Answer from the drawing. Dimensions are ordinates in mm from the lowest x, y and z of the part. A direction names the side the tool comes from. Give positions to 0.01 mm unless a question says otherwise; leave off trailing zeros. Write each loop counter-clockwise with the first axis right and the second up, starting at its lowest first coordinate (ties: lowest second). Pieces come first, ordered by that corner, then holes.
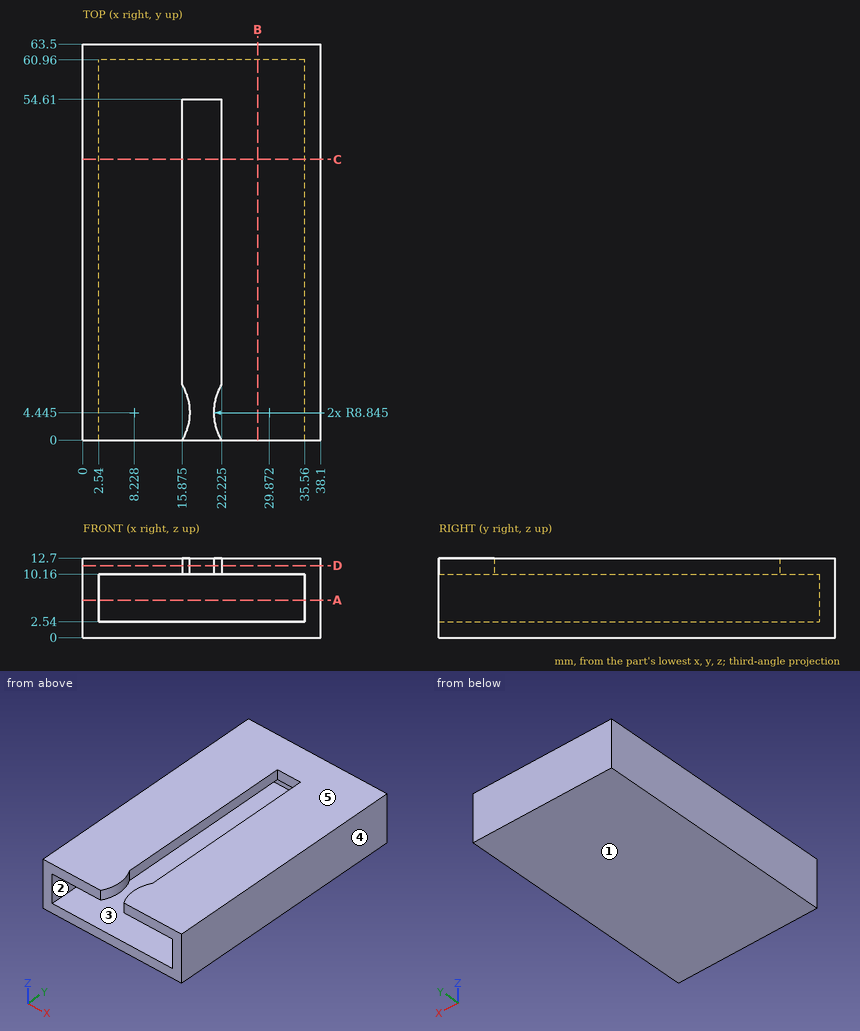
Item 1: Which of the six approach directions +Z, -Z, +X, -X, +Y, -Y give full straight-line access (tool end or side, diameter ignored) to the marked faces 1 and 2?
Result set:
face 1: -Z, +X, -X, +Y, -Y
face 2: -Y
Item 2: Section D-D (z = 11.5) is taken. Write down the section's boundary in (x, y) (1 decimal), and give its area (3 significant figures).
Result set:
outline: (0, 0) - (15.9, 0) arc R8.8 ccw to (15.9, 8.9) - (15.9, 54.6) - (22.2, 54.6) - (22.2, 8.9) arc R8.8 ccw to (22.2, 0) - (38.1, 0) - (38.1, 63.5) - (0, 63.5) - close
area: 2,090 mm2
Item 3: Each of these flat-tipped pins is pushed along its axis until it touches: pin 1 Ø1.3 at (x, z) = (18.5, 11.5) entering from -Y; pin 2 Ø6 at (x, z) = (30.5, 6) entering from -Y. Where does it stop, or does it pass through?
Result set:
pin 1: stops at y = 54.61
pin 2: stops at y = 60.96
Item 4: Determine the mould class of the marked faces 3, 4 and 5 for opening direction Z: pulls with the +Z half, pulls with the -Z half, needs draft (parallel to the pull), parting line crosses it, or undercut.
Result set:
face 3: undercut
face 4: needs draft
face 5: pulls with the +Z half
Item 5: Section B-B (x = 28) is taken. Write down the section's boundary in (y, z).
Result set:
outline: (0, 0) - (63.5, 0) - (63.5, 12.7) - (0, 12.7) - (0, 10.16) - (60.96, 10.16) - (60.96, 2.54) - (0, 2.54) - close
Item 6: Section A-A (z = 6) is taken. Write down the section's boundary in (x, y).
Result set:
outline: (0, 0) - (2.54, 0) - (2.54, 60.96) - (35.56, 60.96) - (35.56, 0) - (38.1, 0) - (38.1, 63.5) - (0, 63.5) - close
Item 7: Find the intervals of material crossed by line 1 along Z through (x, y) = (14.5, 40); line 2 along X through (y, z) = (19, 9); line 3 along X through (y, z) = (52, 11.5) (3 decimals), in increasing order.
Result set:
line 1: z = 0 to 2.54, 10.16 to 12.7
line 2: x = 0 to 2.54, 35.56 to 38.1
line 3: x = 0 to 15.875, 22.225 to 38.1
Item 8: Section C-C (y = 45) is taken. Write down the section's boundary in (x, z) (3 decimals), and give its area (3 significant figures).
Result set:
outline: (0, 0) - (38.1, 0) - (38.1, 12.7) - (22.225, 12.7) - (22.225, 10.16) - (35.56, 10.16) - (35.56, 2.54) - (2.54, 2.54) - (2.54, 10.16) - (15.875, 10.16) - (15.875, 12.7) - (0, 12.7) - close
area: 216 mm2
